from build123d import *

# Parameters (mm, degrees)
F1_DEPTH = 24.13
F3_DEPTH = 25.4
F4_D     = 5
F4_DEPTH = 15.6972
F4_TIP   = 1.5021515476
F6_DEPTH = 3.175
F9_DEPTH = 25.4


# Not quite as in the source:
# - a feature names something its author has since deleted; it is built from what else it names


with BuildPart() as f1:
    # F0 (on Top) → F1 (new body)
    with BuildSketch(Plane.XY):
        with BuildLine():
            Line((-22.0673531294, -31.75), (-22.0673531294, 31.75))
            Line((-22.0673531294, 31.75), (-24.2402065279, 31.75))
            ThreePointArc((-24.2402065279, 31.75), (-37.5816867945, 0), (-24.2402065279, -31.75))
            Line((-24.2402065279, -31.75), (-22.0673531294, -31.75))
        make_face()
    extrude(amount=F1_DEPTH)

    # F2 (on face) → F3 (cut)
    with BuildSketch(Plane.YZ.offset(-22.0673531294)):
        with BuildLine():
            ThreePointArc((-27.7153407028, 16.5054662391), (-27.8542875294, 14.287165191), (-27.90063, 12.065))
            Line((-27.90063, 12.065), (-22.89937, 12.065))
            ThreePointArc((-22.89937, 12.065), (-22.8573758972, 14.078656851), (-22.7314666127, 16.0888121361))
            ThreePointArc((-22.7314666127, 16.0888121361), (-25.0150766063, 18.7890762326), (-27.7153407028, 16.5054662391))
        make_face()
        with BuildLine():
            Line((-22.89937, 12.065), (-27.90063, 12.065))
            ThreePointArc((-27.90063, 12.065), (-27.8542875294, 9.842834809), (-27.7153407028, 7.6245337609))
            ThreePointArc((-27.7153407028, 7.6245337609), (-25.0150766063, 5.3409237674), (-22.7314666127, 8.0411878639))
            ThreePointArc((-22.7314666127, 8.0411878639), (-22.8573758972, 10.051343149), (-22.89937, 12.065))
        make_face()
    extrude(amount=-F3_DEPTH, mode=Mode.SUBTRACT)

    # F4
    with Locations(Plane.YZ.offset(-22.0673531294)):
        with Locations((25.4, 12.065)):
            Hole(F4_D / 2, depth=F4_DEPTH)
            with Locations((0, 0, -(F4_DEPTH + F4_TIP / 2))):  # 118° drill point
                Cone(0, F4_D / 2, F4_TIP, mode=Mode.SUBTRACT)

    # F5 (on face) → F6 (join)
    with BuildSketch(Plane.YZ.offset(-22.0673531294)):
        Polygon((18.8468, 24.13), (-20.2196036578, 24.13), (-20.2196036578, 12.065), (20.3962, 12.065), (20.3962, 24.13), align=None)
        Polygon((20.3962, 12.065), (-20.2196036578, 12.065), (-20.2196036578, 0), (18.8468, 0), (20.3962, 0), align=None)
    extrude(amount=F6_DEPTH)

    # F8 (on offset) → F9 (cut)
    with BuildSketch(Plane.XY.offset(24.13)):
        with BuildLine():
            Line((-27.1383672688, -22.098), (-25.0180043274, -22.098))
            ThreePointArc((-25.0180043274, -22.098), (-24.5480249582, -21.9033281712), (-24.3533531294, -21.433348802))
            Line((-24.3533531294, -21.433348802), (-24.3533531294, -19.1001488633))
            ThreePointArc((-24.3533531294, -19.1001488633), (-24.0116799492, -18.2752768379), (-23.1868079238, -17.9336036578))
            Line((-23.1868079238, -17.9336036578), (-22.344898335, -17.9336036578))
            ThreePointArc((-22.344898335, -17.9336036578), (-21.5200263095, -17.5919304776), (-21.1783531294, -16.7670584522))
            Line((-21.1783531294, -16.7670584522), (-21.1783531294, 16.9436547944))
            ThreePointArc((-21.1783531294, 16.9436547944), (-21.5200263095, 17.7685268198), (-22.344898335, 18.1102))
            Line((-22.344898335, 18.1102), (-23.1868079238, 18.1102))
            ThreePointArc((-23.1868079238, 18.1102), (-24.0116799492, 18.4518731802), (-24.3533531294, 19.2767452056))
            Line((-24.3533531294, 19.2767452056), (-24.3533531294, 21.4333486842))
            ThreePointArc((-24.3533531294, 21.4333486842), (-24.5480249927, 21.9033281367), (-25.0180044452, 22.098))
            Line((-25.0180044452, 22.098), (-27.1383672685, 22.098))
            ThreePointArc((-27.1383672685, 22.098), (-28.9437022551, 21.6431252713), (-30.3179604636, 20.3871157933))
            ThreePointArc((-30.3179604636, 20.3871157933), (-30.4349971545, 20.1980605736), (-30.540806063, 20.0025))
            ThreePointArc((-30.540806063, 20.0025), (-35.2956867945, 0), (-30.5408060633, -20.0025))
            ThreePointArc((-30.5408060633, -20.0025), (-30.4797145494, -20.1187097942), (-30.414655411, -20.2327457441))
            ThreePointArc((-30.414655411, -20.2327457441), (-29.0233896447, -21.5990105168), (-27.1383672688, -22.098))
        make_face()
    extrude(amount=-F9_DEPTH, mode=Mode.SUBTRACT)


solid = f1.part
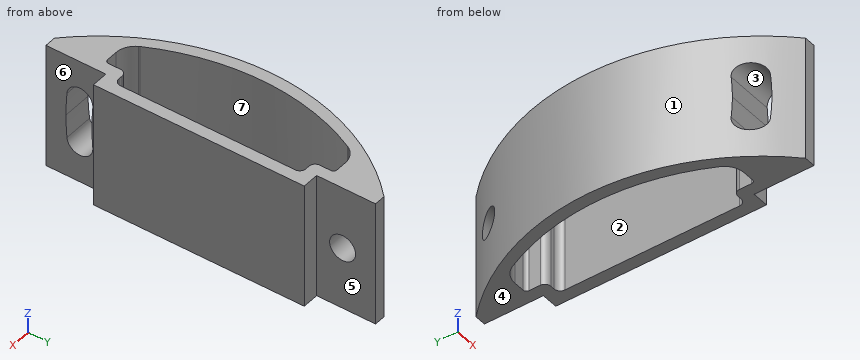
Can you work these out from the model? Positions are in its coordinate system, mm. Face numbers are marked on the shaded views. A direction names the side the tool comes from. Coordinates: 2 decimals unless noted, no trailing zeros. Write each loop counter-clockwise with the first axis right and the second up, starting at its lowest first coordinate (ties: lowest second). Pieces come first, ordered by that corner, then holes. Notation, with made-up numbers: (19.5, 65) - (39.5, 65) arc R12 ccw to (39.5, 70) - close; hole circle Ø9 at (13.5, -2.75). An arc over 180 degrees is marked (long way). Return JSON: item names as keys, results as strings. Group by question number.
Item 1: Please list where these lines run through material, in increasing order: probe 1 along Z at (x, y) = (-24.75, 25.4) (3 decimals); probe 2 along Y at (x, z) = (-24.75, 16.5); probe 3 along Y at (x, z) = (-26, 18.5).
Item 2: If we section it at B-B (y = 24): Write out the boundary of the cut face in (x, z), then the cut area to 3 significant figures.
Item 3: If we section it at D-D (z = 2.25): Write out the boundary of the cut face in (x, y), then the cut area to 3 significant figures.
Item 4: I'm going to push flat-ended pins straight in: pin 1 Ø1.1 at (x, z) = (-26.5, 10) entering from +Y; pin 2 Ø3 at (x, z) = (-30, 15) entering from -Y; pin 3 Ø4 at (y, z) = (25.4, 12.065) entering from +X; pin 4 Ø5 at (x, z) = (-31, 8) entering from -Y. Where does each tip first touch, or does it pass through?
Item 5: Which directions (+Z, -Z, +X, -X, +Y, -Y) give clear straight access to the entire face, cutting with the end or side of a thin tool? Please do the marked faces 5, 6 and 7.
Item 6: If we section it at A-A (z = 9): Write out the boundary of the cut face in (x, y).
Item 7: If we section it at C-C (x = -26): Write out the boundary of the cut face in (y, z) (3 decimals).
Item 8: We'd pull the mould along Y, two halves only. Please class the marked faces 1, 2, 3 and 4: pulls with the +Y half, pulls with the -Y half, needs draft (parallel to the pull), parting line crosses it, or undercut.
Return value:
{
 "1": {"probe 1": "z = 0 to 9.565, 14.565 to 24.13", "probe 2": "y = -31.24 to -27.72, -22.73 to -22.04, 22.04 to 31.24", "probe 3": "y = -29.92 to -26.41, -24.04 to -22.1, 22.1 to 29.92"},
 "2": {"outline": "(-30.55, 0) - (-22.07, 0) - (-22.07, 9.99) - (-30.55, 9.99) - close; (-30.55, 14.14) - (-22.07, 14.14) - (-22.07, 24.13) - (-30.55, 24.13) - close", "area": "169 mm^2"},
 "3": {"outline": "(-24.24, -31.75) - (-22.07, -31.75) - (-22.07, -20.22) - (-18.89, -20.22) - (-18.89, 20.4) - (-22.07, 20.4) - (-22.07, 31.75) - (-24.24, 31.75) arc R44.45 ccw to start; hole (-30.54, -20) arc R3.81 ccw to (-27.14, -22.1) - (-25.02, -22.1) arc R0.66 ccw to (-24.35, -21.43) - (-24.35, -19.1) arc R1.17 cw to (-23.19, -17.93) - (-22.34, -17.93) arc R1.17 ccw to (-21.18, -16.77) - (-21.18, 16.94) arc R1.17 ccw to (-22.34, 18.11) - (-23.19, 18.11) arc R1.17 cw to (-24.35, 19.28) - (-24.35, 21.43) arc R0.66 ccw to (-25.02, 22.1) - (-27.14, 22.1) arc R3.81 ccw to (-30.54, 20) arc R44.45 ccw to start", "area": "339 mm^2"},
 "4": {"pin 1": "stops at y = 29.98", "pin 2": "stops at y = -22.88", "pin 3": "passes through", "pin 4": "stops at y = -24.17"},
 "5": {"face 5": "+Z, -Z, +X, +Y", "face 6": "+Z, -Z, +X, -Y", "face 7": "+Z, -Z"},
 "6": {"outline": "(-31.29, -22.8) - (-22.07, -22.8) - (-22.07, -20.22) - (-18.89, -20.22) - (-18.89, 20.4) - (-22.07, 20.4) - (-22.07, 31.75) - (-24.24, 31.75) arc R44.45 ccw to start; (-27.81, -27.81) arc R44.45 ccw to (-24.24, -31.75) - (-22.07, -31.75) - (-22.07, -27.81) - close; hole (-30.54, -20) arc R3.81 ccw to (-27.14, -22.1) - (-25.02, -22.1) arc R0.66 ccw to (-24.35, -21.43) - (-24.35, -19.1) arc R1.17 cw to (-23.19, -17.93) - (-22.34, -17.93) arc R1.17 ccw to (-21.18, -16.77) - (-21.18, 16.94) arc R1.17 ccw to (-22.34, 18.11) - (-23.19, 18.11) arc R1.17 cw to (-24.35, 19.28) - (-24.35, 21.43) arc R0.66 ccw to (-25.02, 22.1) - (-27.14, 22.1) arc R3.81 ccw to (-30.54, 20) arc R44.45 ccw to start"},
 "7": {"outline": "(-29.925, 0) - (-22.098, 0) - (-22.098, 24.13) - (-29.925, 24.13) - close; (22.098, 0) - (29.925, 0) - (29.925, 24.13) - (22.098, 24.13) - close; hole (-27.715, 7.625) arc R2.501 ccw to (-22.731, 8.041) arc R48.299 cw to (-22.731, 16.089) arc R2.501 ccw to (-27.715, 16.505) arc R53.301 ccw to start; hole circle Ø5 at (25.4, 12.065)"},
 "8": {"face 1": "parting line crosses it", "face 2": "undercut", "face 3": "undercut", "face 4": "needs draft"}
}
